from build123d import *

# Parameters (mm, degrees)
F0_W     = 88.9
F0_H     = 158.75
F1_DEPTH = 63.5
F2_W     = 22.86
F2_H     = 14.4977445151
F2_H_2   = 79.4822554849
F3_DEPTH = 57.15


with BuildPart() as f1:
    # F0 (on Top) → F1 (new body)
    with BuildSketch(Plane.XY):
        with Locations((-17.5175424735, 7.864119485)):
            Rectangle(F0_W, F0_H)
    extrude(amount=F1_DEPTH)

    # F2 (on face) → F3 (cut)
    with BuildSketch(Plane.XY.offset(63.5)):
        Polygon((-16.525246546, 73.9238959342), (-16.525246546, 40.9038959342), (6.334753454, 40.9038959342), (6.334753454, 26.4061514191), (17.7769116252, 26.4061514191), align=None)
        Polygon((-39.385246546, 26.4061514191), (-39.385246546, 40.9038959342), (-16.525246546, 40.9038959342), (-16.525246546, 73.9238959342), (-50.9065217465, 26.4061514191), align=None)
        with Locations((-27.955246546, 33.6550236767)):
            Rectangle(F2_W, F2_H)
        with Locations((-5.095246546, 33.6550236767)):
            Rectangle(F2_W, F2_H)
        with Locations((-5.095246546, -13.3349763233)):
            Rectangle(F2_W, F2_H_2)
        Polygon((17.7769116252, 26.4061514191), (6.334753454, 26.4061514191), (6.334753454, -53.0761040658), align=None)
        with Locations((-27.955246546, -13.3349763233)):
            Rectangle(F2_W, F2_H_2)
        Polygon((-39.385246546, -53.0761040658), (-39.385246546, 26.4061514191), (-50.9065217465, 26.4061514191), align=None)
    extrude(amount=-F3_DEPTH, mode=Mode.SUBTRACT)


solid = f1.part
Could you check a few things on this model? Use its own coordinates, in mm. A direction names the side the tool comes from. Coordinates: 2 decimals unless noted, no trailing zeros. Order: outer loops, then holes, each group sorted by start corner. A loop starts at its lowest first (then second) coordinate and runs counter-clockwise, first axis right, second up.
Q1. Will this pin go through, and if not, where does the flat tip stop? pin 1 (20.5 mm diameter, centred on x = -2, y = 3, fed in from +Z).
Q2. Suppose I cut it at A-A on z = 46.5. Please give me the cut outline in (x, y), and give its area (3 significant figures).
Q3. Thinking about a two-plate mould opening in X: for faces 3 (the flat face through (-33.475, 50.498, 35.325)), 4 (the flat face through (-61.968, 7, 31)), 5 (the flat face through (-18, 9, 0)), which applies, released by +X, released by -X, zero draft, split by the parting line, or undercut?
Q4. Suppose I cut it at C-C on x = -3.5. Please give me the cut outline in (y, z), and give its area (3 significant figures).
Q5. Please list where these lines run through material, in increasing order: L1, parallel to Z at x = -3.5, y = 20; L2, parallel to Y at x = -32.5, z = 49.5; L3, parallel to X at y = 3, z = 35.5.
Q6. Suppose I cut it at B-B on y = 65.5. Please give me the cut outline in (x, z).
Q7. Which directions (+Z, -Z, +X, -X, +Y, -Y) give clear straight access to the entire face, cutting with the end or side of a thin tool? Please do faces 1 (the flat face through (0.87, 49.83, 35.33)), 2 (the flat face through (-18, -71.511, 31)).
Answer:
1. pin 1: stops at z = 6.35
2. outline: (-61.97, -71.51) - (26.93, -71.51) - (26.93, 87.24) - (-61.97, 87.24) - close; hole (-50.91, 26.41) - (-39.39, -53.08) - (6.33, -53.08) - (17.78, 26.41) - (-16.53, 73.92) - close
2. area: 7,930 mm2
3. face 3: undercut
3. face 4: released by -X
3. face 5: zero draft
4. outline: (-71.51, 0) - (87.24, 0) - (87.24, 63.5) - (55.88, 63.5) - (55.88, 6.35) - (-53.08, 6.35) - (-53.08, 63.5) - (-71.51, 63.5) - close
4. area: 3,850 mm2
5. L1: z = 0 to 6.35
5. L2: y = -71.51 to -53.08, 51.85 to 87.24
5. L3: x = -61.97 to -47.51, 14.41 to 26.93
6. outline: (-61.97, 0) - (26.93, 0) - (26.93, 63.5) - (-10.44, 63.5) - (-10.44, 6.35) - (-22.62, 6.35) - (-22.62, 63.5) - (-61.97, 63.5) - close
7. face 1: +Z
7. face 2: +Z, -Z, +X, -X, -Y
